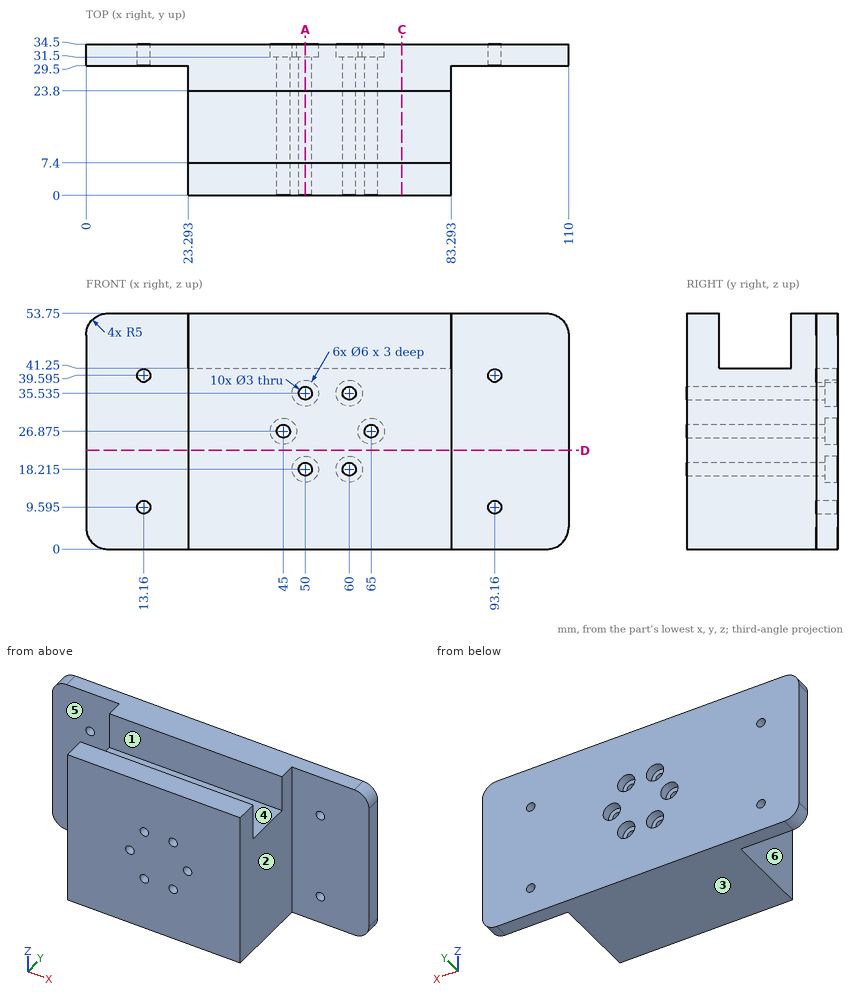
Study the drawing (mm; zero at the part's minimum x, y, z) and answer. A direction names the side the tool comes from. Round coordinates to 2 decimals unless told otherwise and drop trailing zeros. Write each loop counter-clockwise with the first axis right and the second up, starting at its lowest first coordinate (ties: lowest second). Pieces come first, ordered by that corner, then holes. Notation, with made-up numbers: (69.5, 2.5) - (116.5, 2.5) arc R31 cw to (116.5, 30.5) - close; hole circle Ø10 at (43, 62). An arc over 180 degrees is marked (long way). Use a Markdown table: item, result. Add a question column.
1. Consider line 1 (Y direction, x = 33, z = 44.5); line 2 (X direction, y = 16, z = 26); line 3 (Y direction, x = 85.5, z = 19.5). Determine where each line is inside the solid, lowest interval first.
2. Flat-ended cylindrical pins translate along their axes: P1, Ø5, axis at x = 50, z = 18.21, coming from the +Y side; P2, Ø1.5, axis at x = 77.5, y = 12, coming from the +Z side; P3, Ø1, axis at y = 12, z = 22, coming from the +X side; P4, Ø1.8, axis at x = 65, z = 26.875, coming from the -Y side. Find the tip coordinate at first contact, or state that the pin passes through.
3. The part is cut by section A-A (x = 50). Give the number of separate pieces and of enclosed holes in the cut face, and give its area (3 significant figures).
4. A tool of negligible diameter and unlimited length cuts with its end or side. For the marked faces 1, 2 and 3, from which of +Z, -Z, +X, -X, +Y, -Y can it reach the whole face along a straight path? Write none if from no direction.
5. The part is cut by section C-C (x = 72). Write down the section's boundary in (y, z), and give its area (3 significant figures).
6. The part is cut by section D-D (z = 22.5). Write down the section's boundary in (x, y), and give its area (3 significant figures).
7. For a pull along Y with two mould halves and no side action, classify the marked faces 4, 5 and 6 as +Y half, -Y half, draft (parallel to the pull), parting line (faces both ways), or undercut.
Reported:
| question | item | result |
|---|---|---|
| 1 | line 1 | 0 to 7.4, 23.8 to 34.5 |
| 1 | line 2 | 23.29 to 43.78, 46.22 to 63.78, 66.22 to 83.29 |
| 1 | line 3 | 29.5 to 34.5 |
| 2 | P1 | y = 31.5 |
| 2 | P2 | z = 41.25 |
| 2 | P3 | x = 83.29 |
| 2 | P4 | through |
| 3 | separate pieces | 3 |
| 3 | enclosed holes | 0 |
| 3 | area | 1,420 mm^2 |
| 4 | face 1 | +Z, +X, -X |
| 4 | face 2 | +Z, -Z, +X, -Y |
| 4 | face 3 | -Z, +X, -X, +Y, -Y |
| 5 | outline | (0, 0) - (34.5, 0) - (34.5, 53.75) - (23.8, 53.75) - (23.8, 41.25) - (7.4, 41.25) - (7.4, 53.75) - (0, 53.75) - close |
| 5 | area | 1,650 mm^2 |
| 6 | outline | (0, 29.5) - (23.29, 29.5) - (23.29, 0) - (83.29, 0) - (83.29, 29.5) - (110, 29.5) - (110, 34.5) - (0, 34.5) - close |
| 6 | area | 2,320 mm^2 |
| 7 | face 4 | undercut |
| 7 | face 5 | -Y half |
| 7 | face 6 | draft |
